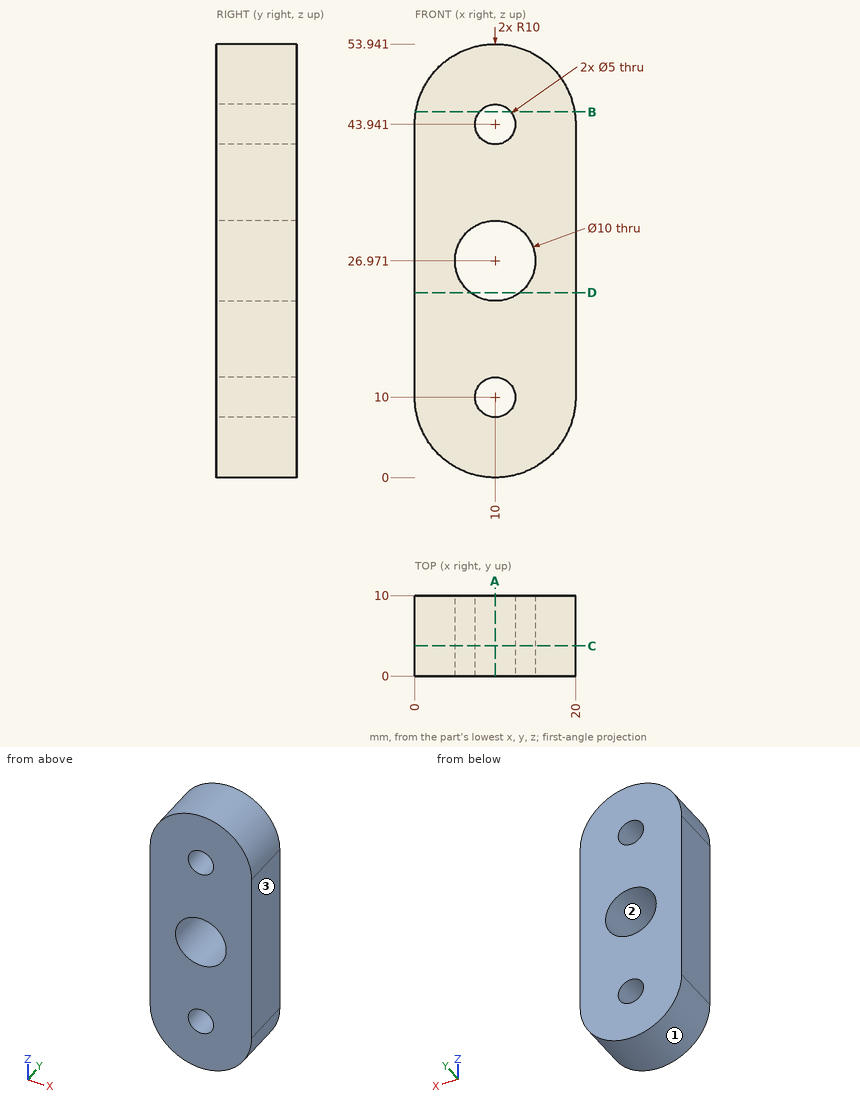
Geometry check sheet. Reference: drawing and pictorial views, mm from the part's lowest x, y, z. Round coordinates to 2 decimals unless told otherwise and drop trailing zeros. Loops run counter-clockwise (first coordinate to the right, second up) from the corner with the lowest first, then second, coordinate; pieces in that order, holes last. Notation, with made-up numbers: (21, 30.25) - (44, 30.25) arc R27 ccw to (44, 53.25) - close; hole circle Ø5 at (40, -23.5). An arc over 180 degrees is marked (long way). One line per question, with ' | ' between items. Start each with the question number.
1. Draft check along Z on the marked faces 1, 2 and 3. Enter one of: released by +Z, released by -Z, zero draft, split by the parting line, or undercut.
2. Depth check by flat-ended pin: pin 1 (5 mm diameter, centred on y = 8, z = 6.5, fed in from -X); pin 2 (1 mm diameter, centred on x = 8.5, y = 2.5, fed in from +Z); pin 3 (5 mm diameter, centred on x = 14, y = 2, fed in from +Z). Enter the tip coordinate at first touch or a pass-through.
3. Cross-section at A-A on x = 10. Record the cut outline in (y, z).
4. Cross-section at D-D on z = 23. Record the cut outline in (x, y).
5. Scan lines: line 1 (Z direction, x = 9.75, y = 5.25) (1 decimal); line 2 (Z direction, x = 10, y = 7); line 3 (Z direction, x = 6.75, y = 4.25) (1 decimal). Record each from-to range of solid material in increasing order. Write a range as [from, to].
6. Cross-section at B-B on z = 45.5. Record the cut outline in (x, y) (1 decimal).
7. Cross-section at C-C on y = 3.75. Record the cut outline in (x, z).
Taken from the geometry:
1) face 1: released by -Z | face 2: undercut | face 3: zero draft
2) pin 1: x = 0.05 | pin 2: z = 53.89 | pin 3: z = 53.83
3) outline: (0, 0) - (10, 0) - (10, 7.5) - (0, 7.5) - close; (0, 12.5) - (10, 12.5) - (10, 21.97) - (0, 21.97) - close; (0, 31.97) - (10, 31.97) - (10, 41.44) - (0, 41.44) - close; (0, 46.44) - (10, 46.44) - (10, 53.94) - (0, 53.94) - close
4) outline: (0, 0) - (6.96, 0) - (6.96, 10) - (0, 10) - close; (13.04, 0) - (20, 0) - (20, 10) - (13.04, 10) - close
5) line 1: [0, 7.5], [12.5, 22], [32, 41.5], [46.4, 53.9] | line 2: [0, 7.5], [12.5, 21.97], [31.97, 41.44], [46.44, 53.94] | line 3: [0.5, 23.2], [30.8, 53.4]
6) outline: (0.1, 0) - (8, 0) - (8, 10) - (0.1, 10) - close; (12, 0) - (19.9, 0) - (19.9, 10) - (12, 10) - close
7) outline: (0, 10) arc R10 ccw to (20, 10) - (20, 43.94) arc R10 ccw to (0, 43.94) - close; hole circle Ø10 at (10, 26.97); hole circle Ø5 at (10, 10); hole circle Ø5 at (10, 43.94)
